Input: part model. Units: mm. Frame: model coordinates. Face numbers are marked on the shaded views. Give positions to 0.01 mm unless a question says otherwise; leave off trailing zeros. Write each loop counter-clockwise with the first axis right and the second up, starting at its lowest first coordinate (ties: lowest second). Pieces come first, ordered by that corner, then holes. Notation, with made-up numbers: (81.5, 42.25) - (100.5, 42.25) arc R20 ccw to (100.5, 79.25) - close; hole circle Ø1 at (28, 42.25). An arc over 180 degrees is marked (long way). Answer as CSV lines item,"result".
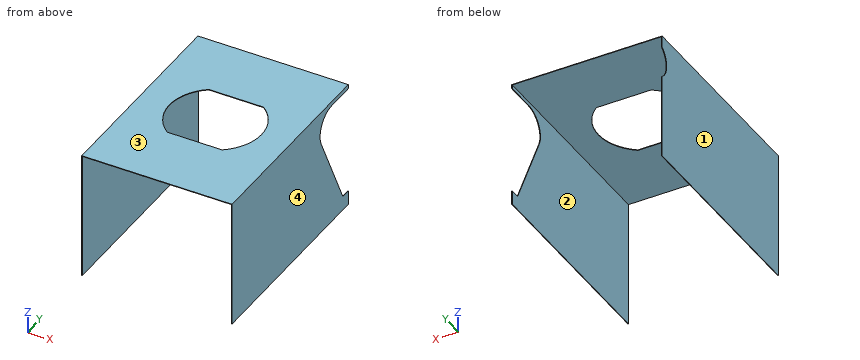
```python
from build123d import *

# Parameters (mm, degrees)
SKETCH1_W            = 69.596
SKETCH1_H            = 96.012
BOSS_EXTRUDE1_DEPTH  = 0.254
SKETCH3_W            = 69.596
SKETCH3_H            = 0.508
BOSS_EXTRUDE2_DEPTH  = 0.254
BOSS_EXTRUDE6_DEPTH  = 0.254
FILLET6_R            = 0.254
SKETCH8_W            = 59.182
SKETCH8_H            = 96.015557392
BOSS_EXTRUDE8_DEPTH  = 0.254
CUT_EXTRUDE1_DEPTH   = 0.254
SKETCH12_W           = 59.182
SKETCH12_H           = 96.012
BOSS_EXTRUDE10_DEPTH = 0.254
SKETCH13_R           = 8.89
CUT_EXTRUDE3_DEPTH   = 0.254
SKETCH24_W           = 13.836349518
SKETCH24_H           = 43.884642402
CUT_EXTRUDE5_DEPTH   = 104.203827287


with BuildPart() as part:
    # Sketch1 → Boss-Extrude1 (new body)
    with BuildSketch(Plane.XY):
        Rectangle(SKETCH1_W, SKETCH1_H)
        with BuildLine():
            Line((12.699364984, -16.764), (-12.699364984, -16.764))
            ThreePointArc((-12.699364984, -16.764), (-21.336, 0.381), (-12.699364984, 17.526))
            Line((-12.699364984, 17.526), (12.699364984, 17.526))
            ThreePointArc((12.699364984, 17.526), (21.336, 0.381), (12.699364984, -16.764))
        make_face(mode=Mode.SUBTRACT)
    extrude(amount=-BOSS_EXTRUDE1_DEPTH)

    # Sketch3 → Boss-Extrude2 (add)
    with BuildSketch(Plane.XY):
        with Locations((0, -17.272)):
            Rectangle(SKETCH3_W, SKETCH3_H)
    extrude(amount=BOSS_EXTRUDE2_DEPTH)

    # Sketch6 → Boss-Extrude6 (add)
    with BuildSketch(Plane.XY):
        with BuildLine():
            Line((14.986, -48.006), (15.24, -48.006))
            ThreePointArc((15.24, -48.006), (0, -32.766), (-15.24, -48.006))
            Line((-15.24, -48.006), (-14.986, -48.006))
            ThreePointArc((-14.986, -48.006), (0, -33.02), (14.986, -48.006))
        make_face()
    extrude(amount=BOSS_EXTRUDE6_DEPTH)

    # Fillet6
    # the kernel refuses this fillet: 0.254 mm, written as the material it takes off along each edge
    with BuildSketch(Plane(origin=(0, -48.006, 0.254), x_dir=(-0.9990995148781596, -0.04242828502574812, 0), z_dir=(0.04242828502574812, -0.9990995148781596, 0))) as fillet6_piece_1:
        with BuildLine():
            CenterArc((14.986 + FILLET6_R, FILLET6_R), FILLET6_R, 180, 90)
            Line((14.986 + FILLET6_R, 0), (14.986, 0))
            Line((14.986, 0), (14.986, FILLET6_R))
        make_face()
    revolve(axis=Axis((0, -48.006, 0.254), (0, 0, -1)), revolution_arc=184.863383217, mode=Mode.SUBTRACT)
    with BuildSketch(Plane(origin=(0, -48.006, 0.254), x_dir=(0.9991292765937022, -0.0417215610128061, 0), z_dir=(-0.0417215610128061, -0.9991292765937022, 0))) as fillet6_piece_2:
        with BuildLine():
            CenterArc((15.24 - FILLET6_R, -FILLET6_R), FILLET6_R, 0, 90)
            Line((15.24 - FILLET6_R, 0), (15.24, 0))
            Line((15.24, 0), (15.24, -FILLET6_R))
        make_face()
    revolve(axis=Axis((0, -48.006, 0.254), (0, 0, 1)), revolution_arc=184.78232683, mode=Mode.SUBTRACT)

    # Sketch8 → Boss-Extrude8 (add)
    with BuildSketch(Plane(origin=(34.798, 0, 0), x_dir=(0, 0, -1), z_dir=(1, 0, 0))):
        with Locations((29.591, 0.001778696)):
            Rectangle(SKETCH8_W, SKETCH8_H)
    extrude(amount=-BOSS_EXTRUDE8_DEPTH)

    # Sketch9 → Cut-Extrude1 (cut)
    with BuildSketch(Plane(origin=(34.798, 0, 0), x_dir=(0, 0, -1), z_dir=(1, 0, 0))):
        with BuildLine():
            Line((2.032, 34.225901784), (2.032, 48.009557392))
            Line((2.032, 48.009557392), (52.578, 48.009557392))
            Line((52.578, 48.009557392), (52.578, 43.536362147))
            Line((52.578, 43.536362147), (15.713824639, 25.655812291))
            ThreePointArc((15.713824639, 25.655812291), (6.500723192, 26.153746568), (2.032, 34.225901784))
        make_face()
    extrude(amount=-CUT_EXTRUDE1_DEPTH, mode=Mode.SUBTRACT)

    # Sketch12 → Boss-Extrude10 (add)
    with BuildSketch(Plane(origin=(-34.798, 0, 0), x_dir=(0, 0, -1), z_dir=(1, 0, 0))):
        with Locations((29.591, 0)):
            Rectangle(SKETCH12_W, SKETCH12_H)
    extrude(amount=BOSS_EXTRUDE10_DEPTH)

    # Sketch13 → Cut-Extrude3 (cut)
    with BuildSketch(Plane.ZY.offset(34.798)):
        with Locations((-12.7, 53.086)):
            Circle(SKETCH13_R)
    extrude(amount=-CUT_EXTRUDE3_DEPTH, mode=Mode.SUBTRACT)

    # Sketch24 → Cut-Extrude5 (cut, through all)
    with BuildSketch(Plane(origin=(34.798, 0, 0), x_dir=(0, 0, -1), z_dir=(1, 0, 0))):
        with Locations((-6.918174759, -26.063678799)):
            Rectangle(SKETCH24_W, SKETCH24_H)
    extrude(amount=-CUT_EXTRUDE5_DEPTH, mode=Mode.SUBTRACT)


solid = part.part
```
Item 1: Cut plane B-B on x = -9.5. Return the cut outline in (y, z).
The answers:
outline,"(-48.01, -0.25) - (-16.76, -0.25) - (-16.76, 0) - (-48.01, 0) - close; (17.53, -0.25) - (48.01, -0.25) - (48.01, 0) - (17.53, 0) - close"
Item 2: Cut plane A-A on y = -3. Return the cut outline in (x, z).
The answers:
outline,"(-34.8, -59.18) - (-34.54, -59.18) - (-34.54, -0.25) - (-21.07, -0.25) - (-21.07, 0) - (-34.8, 0) - close; (21.07, -0.25) - (34.54, -0.25) - (34.54, -59.18) - (34.8, -59.18) - (34.8, 0) - (21.07, 0) - close"
Item 3: Mould query, pull axis X, two halves, no side actions, for the marked faces 1, 2, 3 and 4. Classes: +X half, -X half, draft (parallel to the pull), parting line (faces both ways), or undercut.
The answers:
face 1,"-X half"
face 2,"undercut"
face 3,"draft"
face 4,"+X half"
Item 4: Ray query, line 1 (X direction, y = -33, z = -40); line 2 (Z direction, x = 17.5, y = 36); line 3 (X direction, y = 44.5, z = -25). Return the intervals inside material, ascending. Write a range as from..to.
The answers:
line 1,"-34.8..-34.54, 34.54..34.8"
line 2,"-0.25..0"
line 3,"-34.8..-34.54"
Item 5: Contact query for a flat-ended pin moving along its axis: pin 1 (2 mm diameter, centred on x = -1, y = -22, fed in from -Z). Output: stop coordinate, or through.
The answers:
pin 1,"z = -0.25"
Item 6: Cut plane C-C on z = -48. Return the cut outline in (x, y).
The answers:
outline,"(-34.8, -48.01) - (-34.54, -48.01) - (-34.54, 48.01) - (-34.8, 48.01) - close; (34.54, -48.01) - (34.8, -48.01) - (34.8, 41.32) - (34.54, 41.32) - close"
Item 7: Cut plane D-D on y = -30. Return the cut outline in (x, z), plus the area to 3 significant figures.
The answers:
outline,"(-34.8, -59.18) - (-34.54, -59.18) - (-34.54, -0.25) - (34.54, -0.25) - (34.54, -59.18) - (34.8, -59.18) - (34.8, 0) - (-34.8, 0) - close"
area,"47.6 mm²"
